Check sheet for the modelled part. Datum: model origin and axes. Units: mm. A direction names the side the tool comes from. Coordinates: 2 decimals unless noted, no trailing zeros. Order: outer loops, then holes, each group sorted by start corner. A loop starts at its lowest first (then second) coordinate and runs counter-clockwise, first axis right, second up.
Autodesk Inventor part; units mm, degrees
ref_plane "Work Plane1" through (0, 0, -23.25) normal (0, 0, -1) x (-1, 0, 0)
ref_plane "YZ Plane" through (0, 0, 0) normal (1, 0, 0) x (0, 1, 0)
ref_plane "XZ Plane" through (0, 0, 0) normal (0, 1, 0) x (-1, 0, 0)
sketch "Sketch1" plane through (0, 0, 0) normal (0, 0, 1) x (1, 0, 0)
  circle A0 centre (0, 0) radius 17.875
  dimension "d0" = 35.75
extrude "Extrusion1" add sketch "Sketch1" along normal mid plane 50
fillet "Fillet1" radius 2 1 edges at (-17.875, 0, 25)
shell "Shell1" thickness 0.62 removed faces 1 at (2.0594, 0.4734, -25)
sketch "Sketch2" plane through (0, 0, 25) normal (0, 0, 1) x (1, 0, 0)
  circle A0 centre (0, 0) radius 15.875
  circle A1 centre (0, 0) radius 6.5
  dimension "d5" = 13
extrude "Extrusion2" add sketch "Sketch2" along normal blind 4.5 contours A1
fillet "Fillet2" radius 0.5 2 edges at (-6.5, 0, 25) (-6.5, 0, 29.5)
sketch "Sketch3" plane through (0, 0, 29.5) normal (0, 0, 1) x (1, 0, 0)
  circle A0 centre (0, 0) radius 6
  circle A1 centre (0, 0) radius 1.6
  dimension "d9" = 3.2
extrude "Extrusion3" add sketch "Sketch3" along normal blind 8 contours A1
fillet "Fillet3" radius 1.6 1 edges at (-1.6, 0, 37.5)
sketch "Sketch4" plane through (0, 0, 25) normal (0, 0, 1) x (1, 0, 0)
  circle A0 centre (0, 0) radius 15.875
  point P0 (12.5, 0)
  dimension "d13" = 12.5
hole "Hole1" at (12.5, 0, 25) direction (0, 0, -1) diameter 2.5 depth 8 tip angle 118
mirror "Mirror1" about plane through (0, 0, 0) normal (1, 0, 0) of "Hole1"
ref_plane "Work Plane1" through (0, 0, -23.25) normal (0, 0, -1) x (-1, 0, 0)
sketch "Sketch6" plane through (0, 0, -23.25) normal (0, 0, -1) x (-1, 0, 0)
  circle A0 centre (0, 0) radius 17.255
extrude "Extrusion5" add sketch "Sketch6" against normal blind 0.62
sketch "Sketch7" plane through (0, 0, -23.25) normal (0, 0, -1) x (-1, 0, 0)
  circle A0 centre (0, 0) radius 17.255
  circle A1 centre (0, 0) radius 12
  dimension "d33" = 24
extrude "Extrusion6" add sketch "Sketch7" along normal blind 0.62 contours A1
sketch "Sketch8" plane through (0, 0, -23.87) normal (0, 0, -1) x (-1, 0, 0)
  circle A0 centre (0, 0) radius 12
  circle A1 centre (0, 0) radius 5.375
  dimension "d36" = 10.75
extrude "Extrusion7" add sketch "Sketch8" along normal blind 3 contours A1
sketch "Sketch9" plane through (0, 0, -26.87) normal (0, 0, -1) x (-1, 0, 0)
  circle A0 centre (0, 0) radius 5.375
  circle A1 centre (0, 0) radius 3.45
  dimension "d39" = 6.9
extrude "Extrusion8" cut sketch "Sketch9" against normal blind 0.8 contours A1
sketch "Sketch10" plane through (0, 0, -26.07) normal (0, 0, -1) x (-1, 0, 0)
  circle A0 centre (0, 0) radius 3.45
  circle A1 centre (0, 0) radius 1.6
  dimension "d42" = 3.2
extrude "Extrusion9" add sketch "Sketch10" along normal blind 1 contours A1
sketch "Sketch11" plane through (0, 0, -23.87) normal (0, 0, -1) x (-1, 0, 0)
  circle A0 centre (0, 0) radius 5.375
  circle A1 centre (0, 0) radius 12
  arc A2 (9.2271, 3.15) -> (3.15, 9.2271) centre (0, 0) ccw
  arc A3 (8.1633, 3.15) -> (3.15, 8.1633) centre (0, 0) ccw
  line L0 (3.15, 9.2271) -> (3.15, 8.1633)
  line L1 (8.1633, 3.15) -> (9.2271, 3.15)
  dimension "d45" = 3.15
  dimension "d46" = 3.15
  dimension "d47" = 9.75
  dimension "d48" = 8.75
extrude "Extrusion10" cut sketch "Sketch11" against normal blind 1 contours L1 A3 L0 A2
pattern_circular "Circular Pattern2" count 4 over 360 about axis through (0, 0, 0) along (0, 0, 1) of "Extrusion10"
sketch "Sketch12" plane through (0, 0, -23.25) normal (0, 0, -1) x (-1, 0, 0)
  circle A0 centre (0, 0) radius 12
  circle A1 centre (0, 0) radius 17.255
  line L0 (-14.5, 1.9) -> (-14, 1.9)
  line L1 (-14, 1.9) -> (-14, -1.9)
  line L2 (-14, -1.9) -> (-14.5, -1.9)
  line L3 (-14.5, -1.9) -> (-14.5, 1.9)
  line L4 (0, 0) -> (-16.9017, 0) construction
  point P0 (-14, 0)
  dimension "d54" = 0.5
  dimension "d55" = 3.8
  dimension "d56" = 14
extrude "Extrusion11" add sketch "Sketch12" along normal blind 7.2 contours L0 L1 L2 L3
chamfer "Chamfer1" distance 1 angle 45 2 edges at (14.25, 1.9, -30.45) (14.25, -1.9, -30.45)
sketch "Sketch13" plane through (14.5, -1.9, -23.25) normal (1, 0, 0) x (0, 0, -1)
  line L0 (7.2, 1) -> (7.2, 2.8)
  line L1 (4.2, 1.9) -> (6.2, 3.8) construction
  line L2 (4.2, 1.9) -> (6.2, 0) construction
  dimension "d61" = 3
hole "Hole2" at (14.5, 0, -27.45) direction (-1, 0, 0) diameter 2 depth 1 tip angle 118
mirror "Mirror2" about plane through (0, 0, 0) normal (1, 0, 0) of "Extrusion11", "Chamfer1", "Hole2"
properties part number "RS550 MabuchiMotor" material "Steel, Mild"
(1) Thickness scan on probe 1 along Y at (x, z) = (0, -24.6) (3 decimals); probe 2 along Y at (x, z) = (0, -26.3) (3 decimals); probe 3 along Z at (x, y) = (-4.5, 0.5). Record the ranges inside material, lowest first.
Filled in:
probe 1: y = -17.875 to -17.255, -5.375 to 5.375, 17.255 to 17.875
probe 2: y = -5.375 to -3.45, -1.6 to 1.6, 3.45 to 5.375
probe 3: z = -26.87 to -22.63, 24.38 to 29.5
(2) Cross-section at A-A (z = -11). Enter the section's corners in (x, y) (3 decimals), and give its area (3 significant figures).
Filled in:
outline: circle Ø35.75 at (0, 0); hole circle Ø34.51 at (0, 0)
area: 68.4 mm2
(3) Tool access check on faces 1 (the flat face through (14.5, 0, -26)), 2 (the flat face through (1.25, -1.25, 29.5)), 3 (the cylindrical face through (14.25, -0.04, -26.45)). Record the directions out of +Z, -Z, +X, -X, +Y, -Y that give a thin tool (end or side, any length) a straight path to the whole face; none if there is none.
Filled in:
face 1: -Z
face 2: +Z
face 3: +X
(4) Go/stop test with flat-tipped pins: P1, Ø5, axis at x = 6.5, y = -5, coming from the -Z side; P2, Ø1.5, axis at y = 5, z = 3.5, coming from the +X side; P3, Ø12, axis at x = -11, y = -10.5, coming from the -Z side. Record where each tip stops, or that it passes through.
Filled in:
P1: stops at z = -23.87
P2: stops at x = 17.36
P3: stops at z = -25
(5) Release check for a two-part mould opening along Y. For faces 4 (the cylindrical face through (-5.158, 3.955, 27.226)), 5 (the flat face through (-9, 15, -25)), 6 (the flat face through (-1, 2, -26.07)) record: +Y half, -Y half, draft (parallel to the pull), parting line (faces both ways), or undercut.
Filled in:
face 4: parting line
face 5: draft
face 6: undercut
